Can you work these out from the model? Positions are in its coordinate system, mm. Face numbers are marked on the shaded views. A direction names the side the tool comes from. Give positions to 0.01 mm unless a question says otherwise; leave off trailing zeros. Write each loop counter-clockwise with the first axis right and the second up, starting at its lowest first coordinate (ties: lowest second). Pieces come first, ordered by that corner, then holes.
```python
from build123d import *

# Parameters (mm, degrees)
SKETCH_W   = 30
SKETCH_H   = 30
SKETCH_W_2 = 26
SKETCH_H_2 = 26
PAD_DEPTH  = 500


with BuildPart() as part:
    # Sketch → Pad (new body)
    with BuildSketch(Plane.XZ):
        with Locations((15, 15)):
            Rectangle(SKETCH_W, SKETCH_H)
        with Locations((15, 15)):
            Rectangle(SKETCH_W_2, SKETCH_H_2, mode=Mode.SUBTRACT)
    extrude(amount=PAD_DEPTH)


solid = part.part
```
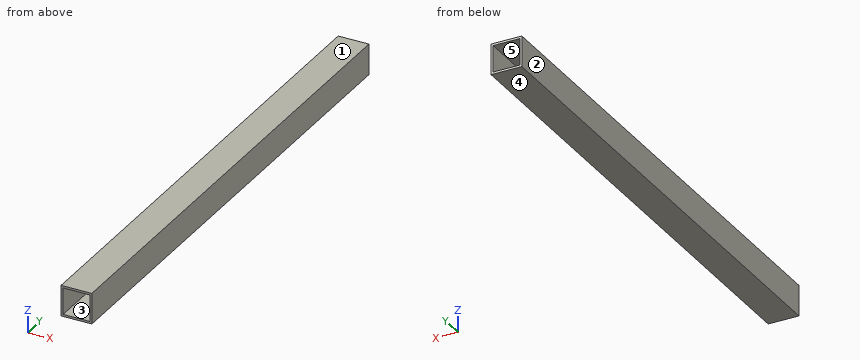
1) Please list where this line runs through material, in increasing order: L1, parallel to X at y = -447.5, z = 27.25.
Values follow:
L1: x = 0 to 2, 28 to 30
2) Suppose I cut it at B-B on x = 10.25. Write out the boundary of the cut face in (y, z).
Values follow:
outline: (-500, 0) - (0, 0) - (0, 2) - (-500, 2) - close; (-500, 28) - (0, 28) - (0, 30) - (-500, 30) - close
3) Suppose I cut it at A-A on z = 20.75. Write out the boundary of the cut face in (x, y), plus the area to 3 significant figures.
Values follow:
outline: (0, -500) - (2, -500) - (2, 0) - (0, 0) - close; (28, -500) - (30, -500) - (30, 0) - (28, 0) - close
area: 2,000 mm2
4) If we mould it in two halves opening along X, with no side actions, what happens to the marked faces 1, 2 and 3? For each: +X half, -X half, draft (parallel to the pull), parting line (faces both ways), or undercut.
Values follow:
face 1: draft
face 2: -X half
face 3: undercut
5) Suppose I cut it at C-C on y = -421.5. Write out the boundary of the cut face in (x, z).
Values follow:
outline: (0, 0) - (30, 0) - (30, 30) - (0, 30) - close; hole (2, 2) - (28, 2) - (28, 28) - (2, 28) - close
6) For the marked faces 4 and 5, which set-ups out of +Z, -Z, +X, -X, +Y, -Y let a thin tool reach every point of the face, with its end or its side?
Values follow:
face 4: -Z, +X, -X, +Y, -Y
face 5: +Y, -Y
